The model under review builds one solid part; all positions refer to its coordinate system, in mm. A direction names the side the tool comes from. Round coordinates to 2 decimals unless told otherwise and drop trailing zeros. Loops run counter-clockwise (first coordinate to the right, second up) from the corner with the lowest first, then second, coordinate; pieces in that order, holes last. Notation, with made-up numbers: (-3, 70) -> (49, 70) arc R19 ccw to (49, 92) -> close; hole circle Ø8 at (-38, 61.25). An arc over 180 degrees is marked (long way). Write each question's results on one line, items separated by ' | '. Start each with the question number.
Item 1: We need section C-C (y = 15). Give the boundary of the cut face in (x, z), and give its area (3 significant figures).
Item 2: We need section B-B (z = -31). Give the boundary of the cut face in (x, y).
Item 3: For L1, parallel to X at y = 19, z = -41.5; L2, parallel to Z at x = -106, y = 86; L3, parallel to Y at x = -115, z = 77, list the stretches that pass through material, from the lowest coordinate up. Write a range as from..to.
Item 4: Clearance check with flat-ended pins moving along their axes: pin 1 Ø10 at (x, z) = (34.5, 75) entering from -Y; pin 2 Ø15 at (y, z) = (-11, 21.5) entering from +X; pin 3 Ø9 at (x, y) = (-16, -13.5) entering from +Z. State where each tip first meets the part, or that it passes through.
Item 5: We need section D-D (z = 61.5). Give the boundary of the cut face in (x, y), and give its area (3 significant figures).
Item 6: Tool access review of faces 1 (the flat face through (-110, -15, 1)), 2 (the flat face through (-110, 54, 1)), 3 (the flat face through (110, -15, -1)): name each direction out of +Z, -Z, +X, -X, +Y, -Y from which nothing blocks a thin tool from reaching the whole face with its end or side.
Item 7: We need section A-A (x = 71.5). Give the boundary of the cut face in (y, z).
Autodesk Inventor part; units mm, degrees
ref_plane "YZ Plane" through (0, 0, 0) normal (1, 0, 0) x (0, 1, 0)
ref_plane "XZ Plane" through (0, 0, 0) normal (0, 1, 0) x (-1, 0, 0)
ref_plane "XY Plane" through (0, 0, 0) normal (0, 0, 1) x (1, 0, 0)
sketch "Sketch1" plane through (0, 0, 0) normal (0, 1, 0) x (-1, 0, 0)
  line L0 (-150, 100) -> (150, 100)
  line L1 (150, 100) -> (150, -100)
  line L2 (150, -100) -> (-150, -100)
  line L3 (-150, -100) -> (-150, 100)
  line L4 (-110, 55) -> (110, 55)
  line L5 (110, 55) -> (110, -55)
  line L6 (110, -55) -> (-110, -55)
  line L7 (-110, -55) -> (-110, 55)
  line L8 (-110, 55) -> (110, -55) construction
  line L9 (110, 55) -> (-110, -55) construction
  point P0 (0, 0)
  dimension "d0" = 300
  dimension "d1" = 200
  dimension "d3" = 220
  dimension "d4" = 110
extrude "Extrusion1" add sketch "Sketch1" along normal blind 10
extrude "Extrusion2" add sketch "Sketch1" along normal blind 100 contours L4 L5 L6 L7
extrude "Extrusion3" add sketch "Sketch1" against normal blind 30 contours L4 L5 L6 L7
Here are the results:
1) outline: (-110, -55) -> (110, -55) -> (110, 55) -> (-110, 55) -> close | area: 24,200 mm2
2) outline: (-150, 0) -> (-110, 0) -> (-110, -30) -> (110, -30) -> (110, 0) -> (150, 0) -> (150, 10) -> (110, 10) -> (110, 100) -> (-110, 100) -> (-110, 10) -> (-150, 10) -> close
3) L1: x = -110..110 | L2: z = -55..55 | L3: y = 0..10
4) pin 1: stops at y = 0 | pin 2: stops at x = 110 | pin 3: stops at z = 55
5) outline: (-150, 0) -> (150, 0) -> (150, 10) -> (-150, 10) -> close | area: 3,000 mm2
6) face 1: +Z, -Z, -X, -Y | face 2: +Z, -Z, -X, +Y | face 3: +Z, -Z, +X, -Y
7) outline: (-30, -55) -> (0, -55) -> (0, -100) -> (10, -100) -> (10, -55) -> (100, -55) -> (100, 55) -> (10, 55) -> (10, 100) -> (0, 100) -> (0, 55) -> (-30, 55) -> close
